Can you work these out from the model? Positions are in its coordinate system, mm. Coordinates: 2 decimals unless noted, no trailing zeros. Order: outer loops, then holes, each group sorted by start corner. A loop starts at its lowest first (then second) coordinate and runs counter-clockwise, first axis right, second up. Notation, with made-up numbers: (46.5, -10) - (93.5, -10) arc R18 cw to (93.5, 18) - close; hole circle Ø1 at (-33, -22). An arc over 180 degrees is marked (long way). Use a Markdown table: item, result. Add a question column.
(1) We'd pull the mould along Y, two halves only. Please class faces 1 (the cylindrical face through (-1.5, 0.07, -0.01)), 2 (the flat face through (0, 4, -1)), 3 (the flat face through (0, -2.5, 0)): pulls with the +Y half, pulls with the -Y half, needs draft (parallel to the pull), parting line crosses it, or undercut.
(2) For pin 1 Ø2.5 at (x, y) = (0, 0) entering from +Z, with a flat end and sliding along its axis, tell me the tip position at first contact or that it passes through.
(3) I want a section at B-B (z = 0). List the corners of the cut face in (x, y) for me.
(4) If I drill on L1, parallel to Y at x = 0, z = -0.6; L2, parallel to Y at x = 1, z = 0.15; L3, parallel to X at y = 1, z = -0.3, over which ranges is the centre line in solid material (lowest first)? Write a range as [from, to].
(5) I want a section at C-C (y = 0). List the corners of the cut face in (x, z) for me.
(6) I want a section at A-A (x = 0). List the corners of the cut face in (y, z) for me.
```python
from build123d import *

# Parameters (mm, degrees)
SKETCH1_R           = 1.5
BOSS_EXTRUDE1_DEPTH = 1


with BuildPart() as part:
    # Sketch1 → Boss-Extrude1 (new, symmetric)
    with BuildSketch(Plane.XY):
        with BuildLine():
            Line((-21, -2.5), (21, -2.5))
            ThreePointArc((21, -2.5), (23.828427125, -1.328427125), (25, 1.5))
            Line((25, 1.5), (25, 9.5))
            Line((25, 9.5), (-25, 9.5))
            Line((-25, 9.5), (-25, 1.5))
            ThreePointArc((-25, 1.5), (-23.828427125, -1.328427125), (-21, -2.5))
        make_face()
        Circle(SKETCH1_R, mode=Mode.SUBTRACT)
    extrude(amount=BOSS_EXTRUDE1_DEPTH, both=True)


solid = part.part
```
Answers follow:
| question | item | result |
|---|---|---|
| 1 | face 1 | undercut |
| 1 | face 2 | needs draft |
| 1 | face 3 | pulls with the -Y half |
| 2 | pin 1 | passes through |
| 3 | outline | (-25, 1.5) arc R4 ccw to (-21, -2.5) - (21, -2.5) arc R4 ccw to (25, 1.5) - (25, 9.5) - (-25, 9.5) - close; hole circle Ø3 at (0, 0) |
| 4 | L1 | y = [-2.5, -1.5], [1.5, 9.5] |
| 4 | L2 | y = [-2.5, -1.12], [1.12, 9.5] |
| 4 | L3 | x = [-24.97, -1.12], [1.12, 24.97] |
| 5 | outline | (-24.71, -1) - (-1.5, -1) - (-1.5, 1) - (-24.71, 1) - close; (1.5, -1) - (24.71, -1) - (24.71, 1) - (1.5, 1) - close |
| 6 | outline | (-2.5, -1) - (-1.5, -1) - (-1.5, 1) - (-2.5, 1) - close; (1.5, -1) - (9.5, -1) - (9.5, 1) - (1.5, 1) - close |
